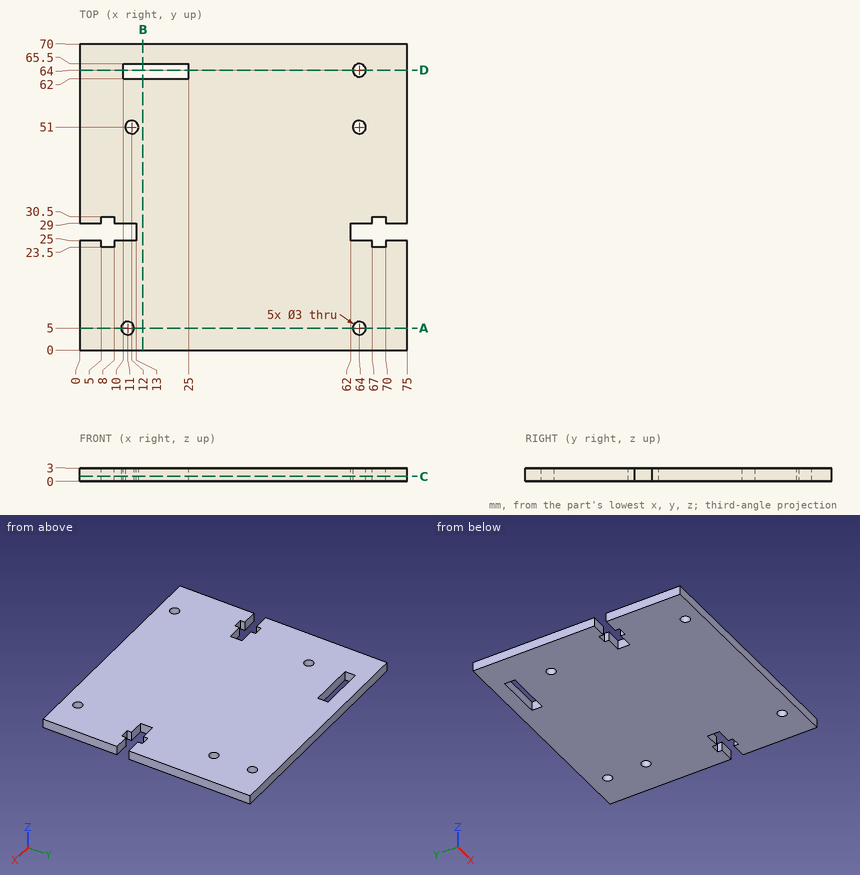
Design review of the part shown in the three views and the two pictorial views. Dimensions are in mm from the part's minimum x, y and z. Round coordinates to 2 decimals unless told otherwise and drop trailing zeros. Loops run counter-clockwise (first coordinate to the right, second up) from the corner with the lowest first, then second, coordinate; pieces in that order, holes last. Notation, with made-up numbers: (77.5, 36) - (117.5, 36) arc R6 ccw to (117.5, 40) - close; hole circle Ø1 at (24.25, -19.75). An arc over 180 degrees is marked (long way). One line per item, written item: value. Start each with the question number.
Item 1: Clearance check with a flat-ended pin moving along its axis: pin 1 Ø1.8 at (x, y) = (64, 64) entering from +Z. State where the tip first meets the part, or that it passes through.
Item 2: Take a section at C-C (z = 1.1). State how many separate pieces and enclosed holes the cut face has, plus the area to 3 significant figures.
Item 3: Take a section at D-D (y = 64). Give the boundary of the cut face in (x, z).
Item 4: Take a section at A-A (y = 5). Give the boundary of the cut face in (x, z).
Item 5: Take a section at B-B (x = 14.5). Give the boundary of the cut face in (y, z).
Item 6: For L1, parallel to X at y = 51, z = 1.45; L2, parallel to Y at x = 64, z = 1.6; L3, parallel to Y at x = 69.5, z = 2.6, list the stretches that pass through material, from the lowest coordinate up.
Answer below:
1. pin 1: passes through
2. separate pieces: 1
2. enclosed holes: 6
2. area: 5,040 mm2
3. outline: (0, 0) - (10, 0) - (10, 3) - (0, 3) - close; (25, 0) - (62.5, 0) - (62.5, 3) - (25, 3) - close; (65.5, 0) - (75, 0) - (75, 3) - (65.5, 3) - close
4. outline: (0, 0) - (9.5, 0) - (9.5, 3) - (0, 3) - close; (12.5, 0) - (62.5, 0) - (62.5, 3) - (12.5, 3) - close; (65.5, 0) - (75, 0) - (75, 3) - (65.5, 3) - close
5. outline: (0, 0) - (62, 0) - (62, 3) - (0, 3) - close; (65.5, 0) - (70, 0) - (70, 3) - (65.5, 3) - close
6. L1: x = 0 to 10.5, 13.5 to 62.5, 65.5 to 75
6. L2: y = 0 to 3.5, 6.5 to 25, 29 to 49.5, 52.5 to 62.5, 65.5 to 70
6. L3: y = 0 to 23.5, 30.5 to 70
